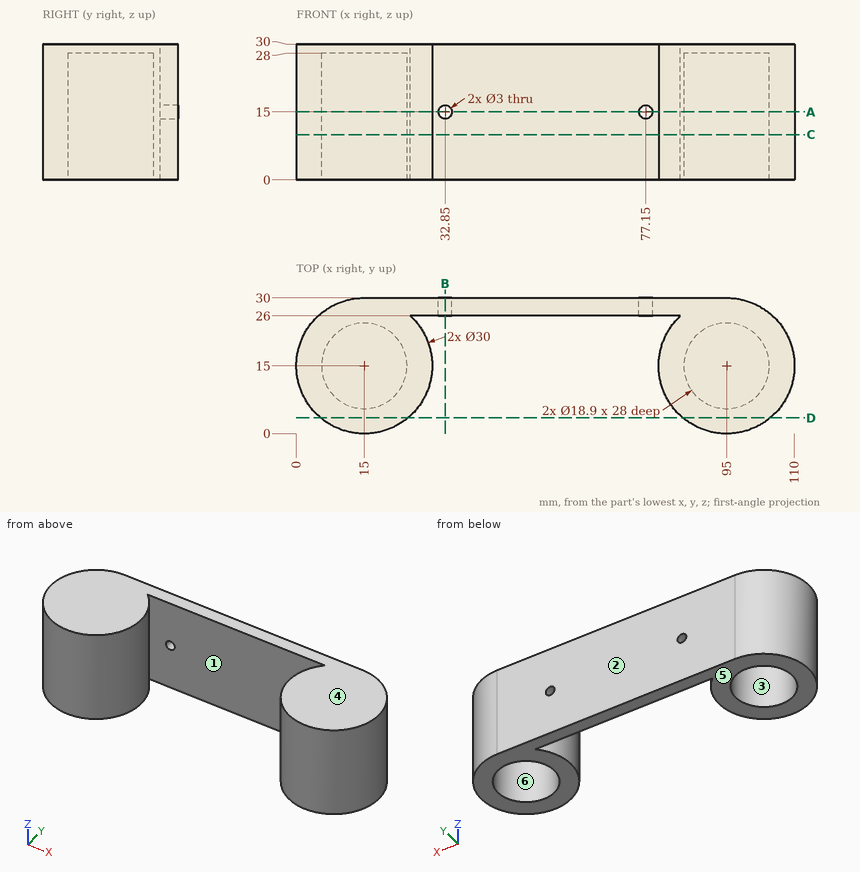
Input: dimensioned drawing with shaded views. Units: mm. Origin: part minimum x, y, z. A direction names the side the tool comes from. Round coordinates to 2 decimals unless told otherwise and drop trailing zeros. Loops run counter-clockwise (first coordinate to the right, second up) from the corner with the lowest first, then second, coordinate; pieces in that order, holes last. Notation, with made-up numbers: M 82.5,75.25 L 100.5,75.25 A30 cw 100.5,99.25 Z; hole C -34.5,14 d6. An arc over 180 degrees is marked long. One line per question, with ' | ' between items.
(1) Cut plane C-C on z = 10. Return the cut outline in (x, y), plus the area to 3 significant figures.
Check result:
outline: M 15,30 A15 ccw long 25.2,26 L 84.8,26 A15 ccw long 95,30 Z; hole C 15,15 d18.9; hole C 95,15 d18.9 | area: 1,120 mm2
(2) Cut plane A-A on z = 15. Return the cut outline in (x, y), plus the area to 3 significant figures.
Check result:
outline: M 15,30 A15 ccw long 25.2,26 L 31.35,26 L 31.35,30 Z; M 34.35,26 L 75.65,26 L 75.65,30 L 34.35,30 Z; M 78.65,26 L 84.8,26 A15 ccw long 95,30 L 78.65,30 Z; hole C 15,15 d18.9; hole C 95,15 d18.9 | area: 1,090 mm2
(3) Contact query for flat-ended pins moving along their axis: P1, Ø4, axis at x = 28, y = 5, coming from the -Z side; P2, Ø1.5, axis at y = 20.5, z = 25.5, coming from the -X side; P3, Ø2, axis at y = 3, z = 14.5, coming from the +X side; P4, Ø2, axis at y = 20, z = 18.5, coming from the -X side. Output: stop coordinate, or through.
Check result:
P1: stops at z = 0 | P2: stops at x = 0.77 | P3: stops at x = 105.2 | P4: stops at x = 0.54
(4) Cut plane B-B on x = 32.85. Return the cut outline in (y, z).
Check result:
outline: M 26,0 L 30,0 L 30,13.5 L 26,13.5 Z; M 26,16.5 L 30,16.5 L 30,30 L 26,30 Z
(5) Access query for the marked faces 5 and 6. Directions: +Z, -Z, +X, -X, +Y, -Y. A direction counts if a zero-diameter tool reaches every point of the face in a straight line with its end or side. Return the directions, or none.
Check result:
face 5: -Z, +X, -X, +Y, -Y | face 6: -Z
(6) Cut plane D-D on y = 3.5. Return the cut outline in (x, z), plus the area to 3 significant figures.
Check result:
outline: M 5.37,0 L 24.63,0 L 24.63,30 L 5.37,30 Z; M 85.37,0 L 104.63,0 L 104.63,30 L 85.37,30 Z | area: 1,160 mm2
(7) Material intervals for line 1 along X through (y, z) = (14, 21.25); line 2 along X through (y, z) = (9, 5.75); line 3 along X through (y, z) = (26.9, 15), sorted ascending. Write a range as from..to.
Check result:
line 1: x = 0.03..5.6, 24.4..29.97, 80.03..85.6, 104.4..109.97 | line 2: x = 1.25..7.7, 22.3..28.75, 81.25..87.7, 102.3..108.75 | line 3: x = 5.87..31.35, 34.35..75.65, 78.65..104.13
(8) Pull-direction query (Y, two-part tool) for the marked faces 1, 2, 3 and 4; classes: +Y half, -Y half, draft (parallel to the pull), parting line (faces both ways), or undercut.
Check result:
face 1: undercut | face 2: +Y half | face 3: undercut | face 4: draft
